from build123d import *

# Parameters (mm, degrees)
BOSS_EXTRUDE1_DEPTH                                 = 15
CBORE_FOR_M6_HEX_SOCKET_HEAD_CAP_SCREW1_D           = 6.6
CBORE_FOR_M6_HEX_SOCKET_HEAD_CAP_SCREW1_CBORE_D     = 11
CBORE_FOR_M6_HEX_SOCKET_HEAD_CAP_SCREW1_CBORE_DEPTH = 6.4
TAP_DRILL_FOR_M6_TAP1_D                             = 5
CHAMFER1_SIZE                                       = 0.5


with BuildPart() as part:
    # Sketch1 → Boss-Extrude1 (new body)
    with BuildSketch(Plane.XY):
        with BuildLine():
            Line((22.658191436, -18.599539786), (31.14347281, -12.114258412))
            ThreePointArc((31.14347281, -12.114258412), (32.878700441, -10.006041207), (33.5, -7.347172731))
            Line((33.5, -7.347172731), (33.5, 17.167545894))
            ThreePointArc((33.5, 17.167545894), (32.621320344, 19.288866238), (30.5, 20.167545894))
            Line((30.5, 20.167545894), (21.5, 20.167545894))
            ThreePointArc((21.5, 20.167545894), (19.378679656, 19.288866238), (18.5, 17.167545894))
            Line((18.5, 17.167545894), (18.5, -0.347172731))
            ThreePointArc((18.5, -0.347172731), (18.043277195, -2.643273326), (16.742640687, -4.589813418))
            Line((16.742640687, -4.589813418), (16.257359313, -5.075094793))
            ThreePointArc((16.257359313, -5.075094793), (14.31081922, -6.375731301), (12.014718626, -6.832454106))
            Line((12.014718626, -6.832454106), (-30.5, -6.832454106))
            Line((-30.5, -6.832454106), (-30.5, -19.832454106))
            Line((-30.5, -19.832454106), (19.014718626, -19.832454106))
            ThreePointArc((19.014718626, -19.832454106), (20.937930252, -19.51587359), (22.658191436, -18.599539786))
        make_face()
    extrude(amount=BOSS_EXTRUDE1_DEPTH)

    # CBORE for M6 Hex Socket Head Cap Screw1 (through all)
    with Locations(Plane.XY.offset(15)):
        with Locations((26, 12.167545894), (26, -5.832454106)):
            CounterBoreHole(CBORE_FOR_M6_HEX_SOCKET_HEAD_CAP_SCREW1_D / 2, CBORE_FOR_M6_HEX_SOCKET_HEAD_CAP_SCREW1_CBORE_D / 2, CBORE_FOR_M6_HEX_SOCKET_HEAD_CAP_SCREW1_CBORE_DEPTH)

    # Tap Drill for M6 Tap1 (through all)
    with Locations(Plane(origin=(0, -6.832454106, 0), x_dir=(1, 0, 0), z_dir=(0, 1, 0))):
        with Locations((-24, -7.5)):
            Hole(TAP_DRILL_FOR_M6_TAP1_D / 2)

    # Chamfer1
    chamfer1_edges = [part.edges().sort_by_distance(p)[0] for p in [
        (20.937930252, -19.51587359, 15),
        (26.900832123, -15.356899099, 15),
        (32.878700441, -10.006041207, 15),
        (33.5, 4.910186582, 15),
        (32.621320344, 19.288866238, 15),
        (26, 20.167545894, 15),
        (19.378679656, 19.288866238, 15),
        (18.5, 8.410186582, 15),
        (18.043277195, -2.643273326, 15),
        (16.5, -4.832454106, 15),
        (-30.5, -13.332454106, 15),
        (14.31081922, -6.375731301, 15),
        (20.5, -5.832454106, 15),
        (-9.242640687, -6.832454106, 15),
        (20.5, 12.167545894, 15),
        (-5.742640687, -19.832454106, 15),
    ]]
    chamfer(chamfer1_edges, length=CHAMFER1_SIZE)


solid = part.part
Work out the finished part from the listing and answer in its coordinate system (mm). A direction names the side the tool comes from. Give positions to 0.01 mm unless a question says otherwise; leave off trailing zeros. Write each loop counter-clockwise with the first axis right and the second up, starting at its lowest first coordinate (ties: lowest second). Pieces come first, ordered by that corner, then holes.
Q1. A tool of negligible diameter and unlimited length cuts with its end or side. For faces 4 (the face through (32.64, 19.27, 7.15)), 5 (the face through (18.5, 9, 7)), from which of +Z, -Z, +X, -X, +Y, -Y can it reach the whole face along a straight path? Write none if from no direction.
Answer:
face 4: +Z, -Z, +X, +Y
face 5: +Z, -Z, -X, +Y
Q2. The part is cut by section D-D on x = -1. Give the vertices of the cut face in (y, z), and give its area (3 significant figures).
Answer:
outline: (-19.83, 0) - (-6.83, 0) - (-6.83, 14.5) - (-7.33, 15) - (-19.33, 15) - (-19.83, 14.5) - close
area: 195 mm2
Q3. Given pin 1 (1.5 mm diameter, centred on y = 8, z = 7, fed in from -X); pin 2 (1.5 mm diameter, centred on x = 21.5, z = 4, fed in from -Y); pin 3 (5 mm diameter, centred on x = -10, z = 2, fed in from +Y); pin 4 (5 mm diameter, centred on x = -2, y = -2, fed in from +Z), each flat-ended and moving along its own axis, determine where each tip first touches the part or whether it passes through.
Answer:
pin 1: stops at x = 18.5
pin 2: stops at y = -19.58
pin 3: stops at y = -6.83
pin 4: passes through
Q4. The part is cut by section C-C on z = 13.25. Give the vertices of the cut face in (x, y).
Answer:
outline: (-30.5, -19.83) - (19.01, -19.83) arc R6 ccw to (22.66, -18.6) - (31.14, -12.11) arc R6 ccw to (33.5, -7.35) - (33.5, 17.17) arc R3 ccw to (30.5, 20.17) - (21.5, 20.17) arc R3 ccw to (18.5, 17.17) - (18.5, -0.35) arc R6 cw to (16.74, -4.59) - (16.26, -5.08) arc R6 cw to (12.01, -6.83) - (-30.5, -6.83) - close; hole circle Ø11 at (26, -5.83); hole circle Ø11 at (26, 12.17)
Q5. The part is cut by section B-B on z = 7.5. Give the vertices of the cut face in (x, y), and give its area (3 significant figures).
Answer:
outline: (-30.5, -19.83) - (-26.5, -19.83) - (-26.5, -6.83) - (-30.5, -6.83) - close; (-21.5, -19.83) - (19.01, -19.83) arc R6 ccw to (22.66, -18.6) - (31.14, -12.11) arc R6 ccw to (33.5, -7.35) - (33.5, 17.17) arc R3 ccw to (30.5, 20.17) - (21.5, 20.17) arc R3 ccw to (18.5, 17.17) - (18.5, -0.35) arc R6 cw to (16.74, -4.59) - (16.26, -5.08) arc R6 cw to (12.01, -6.83) - (-21.5, -6.83) - close; hole circle Ø6.6 at (26, -5.83); hole circle Ø6.6 at (26, 12.17)
area: 1,050 mm2
Q6. Straight lines are drawn through the part: L1, parallel to Z at x = -24, y = -12; L2, parallel to X at y = 12, z = 2.75; L3, parallel to Z at x = 23.5, y = -3. For each, find the intervals that lie inside material, in ascending order.
Answer:
L1: z = 0 to 5, 10 to 15
L2: x = 18.5 to 22.7, 29.3 to 33.5
L3: z = 0 to 8.6
Q7. For a pull along X with two mould halves and no side action, classify faces 1 (the face through (-9, -6.832, 7)), 2 (the face through (24.8, -11.2, 11.6)), 3 (the face through (14.341, -6.363, 7.148)) as released by +X, released by -X, zero draft, split by the parting line, or undercut.
Answer:
face 1: zero draft
face 2: undercut
face 3: released by -X
Q8. The part is cut by section A-A on x = -24. Give the vertices of the cut face in (y, z).
Answer:
outline: (-19.83, 0) - (-6.83, 0) - (-6.83, 5) - (-19.83, 5) - close; (-19.83, 10) - (-6.83, 10) - (-6.83, 14.5) - (-7.33, 15) - (-19.33, 15) - (-19.83, 14.5) - close
